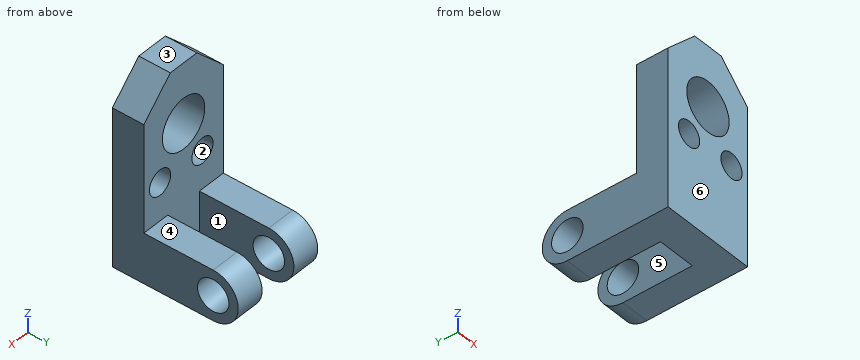
```python
from build123d import *

# Parameters (mm, degrees)
SKETCH2_W           = 30
SKETCH2_H           = 60
BOSS_EXTRUDE1_DEPTH = 10
CHAMFER1_SIZE       = 10
CHAMFER2_SIZE       = 10
SKETCH3_W           = 15.904721494
SKETCH3_H           = 22
BOSS_EXTRUDE2_DEPTH = 9
CUT_EXTRUDE4_REACH  = 56.771
SKETCH5_R           = 8
SKETCH6_R           = 7.952360747
BOSS_EXTRUDE3_DEPTH = 9
CUT_EXTRUDE5_REACH  = 70.795
SKETCH8_R           = 5
CUT_EXTRUDE6_REACH  = 60.421
SKETCH9_R           = 4


with BuildPart() as part:
    # Sketch2 → Boss-Extrude1 (new body)
    with BuildSketch(Plane(origin=(0, 0, 0), x_dir=(1, 0, 0), z_dir=(0, 1, 0))):
        with Locations((-1.70984456, 17.292746114)):
            Rectangle(SKETCH2_W, SKETCH2_H)
    extrude(amount=BOSS_EXTRUDE1_DEPTH)

    # Chamfer1
    chamfer1_edges = [part.edges().sort_by_distance(p)[0] for p in [
        (-16.70984456, 5, 12.707253886),
    ]]
    chamfer(chamfer1_edges, length=CHAMFER1_SIZE)

    # Chamfer2
    chamfer2_edges = [part.edges().sort_by_distance(p)[0] for p in [
        (13.29015544, 5, 12.707253886),
    ]]
    chamfer(chamfer2_edges, length=CHAMFER2_SIZE)

    # Sketch3 → Boss-Extrude2 (add)
    with BuildSketch(Plane(origin=(13.29015544, 0, 0), x_dir=(0, 0, -1), z_dir=(1, 0, 0))):
        with Locations((39.340385367, 21)):
            Rectangle(SKETCH3_W, SKETCH3_H)
    boss_extrude2 = extrude(amount=-BOSS_EXTRUDE2_DEPTH)

    # Sketch5 → Cut-Extrude4 (cut, up to next)
    with BuildSketch(Plane(origin=(0, 10, 0), x_dir=(1, 0, 0), z_dir=(0, 1, 0)), mode=Mode.PRIVATE) as cut_extrude4_sk1:
        with Locations(Location((-1.70984456, 6.38802462, 0), (0, 0, 270))):
            Circle(SKETCH5_R)
    cut_extrude4_tool1 = extrude(cut_extrude4_sk1.sketch, amount=-CUT_EXTRUDE4_REACH, mode=Mode.PRIVATE) & part.part
    add(cut_extrude4_tool1.solids().sort_by_distance((-1.709845, 10, -6.388025))[0], mode=Mode.SUBTRACT)

    # Sketch6 → Boss-Extrude3 (add)
    with BuildSketch(Plane(origin=(13.29015544, 0, 0), x_dir=(0, 0, -1), z_dir=(1, 0, 0))):
        with Locations((39.340385367, 32)):
            Circle(SKETCH6_R)
    boss_extrude3 = extrude(amount=-BOSS_EXTRUDE3_DEPTH)

    # Sketch8 → Cut-Extrude5 (cut, up to next)
    with BuildSketch(Plane(origin=(13.29015544, 0, 0), x_dir=(0, 0, -1), z_dir=(1, 0, 0)), mode=Mode.PRIVATE) as cut_extrude5_sk1:
        with Locations((39.340385367, 32)):
            Circle(SKETCH8_R)
    cut_extrude5_tool1 = extrude(cut_extrude5_sk1.sketch, amount=-CUT_EXTRUDE5_REACH, mode=Mode.PRIVATE) & part.part
    cut_extrude5 = cut_extrude5_tool1.solids().sort_by_distance((13.290155, 32, -39.340385))[0]
    add(cut_extrude5, mode=Mode.SUBTRACT)

    # Mirror6: Boss-Extrude2, Boss-Extrude3, Cut-Extrude5 across plane
    add(boss_extrude2.mirror(Plane.ZY.offset(1.70984456)))
    add(boss_extrude3.mirror(Plane.ZY.offset(1.70984456)))
    add(cut_extrude5.mirror(Plane.ZY.offset(1.70984456)), mode=Mode.SUBTRACT)

    # Sketch9 → Cut-Extrude6 (cut, up to next)
    with BuildSketch(Plane(origin=(0, 10, 0), x_dir=(1, 0, 0), z_dir=(0, 1, 0)), mode=Mode.PRIVATE) as cut_extrude6_sk1:
        with Locations(Location((-8.831623879, 19.34363435, 0), (0, 0, 270))):
            Circle(SKETCH9_R)
    cut_extrude6_tool1 = extrude(cut_extrude6_sk1.sketch, amount=-CUT_EXTRUDE6_REACH, mode=Mode.PRIVATE) & part.part
    # Sketch9 → Cut-Extrude6 (cut, up to next)
    with BuildSketch(Plane(origin=(0, 10, 0), x_dir=(1, 0, 0), z_dir=(0, 1, 0)), mode=Mode.PRIVATE) as cut_extrude6_sk2:
        with Locations(Location((7.168376121, 19.34363435, 0), (0, 0, 270))):
            Circle(SKETCH9_R)
    cut_extrude6_tool2 = extrude(cut_extrude6_sk2.sketch, amount=-CUT_EXTRUDE6_REACH, mode=Mode.PRIVATE) & part.part
    add(cut_extrude6_tool1.solids().sort_by_distance((-8.831624, 10, -19.343634))[0], mode=Mode.SUBTRACT)
    add(cut_extrude6_tool2.solids().sort_by_distance((7.168376, 10, -19.343634))[0], mode=Mode.SUBTRACT)


solid = part.part
```
Design review of the part built by this model. Coordinates are the model's own, in mm. Face numbers are marked on the shaded views. A direction names the side the tool comes from. Give positions to 0.01 mm unless a question says otherwise; leave off trailing zeros. Order: outer loops, then holes, each group sorted by start corner. A loop starts at its lowest first (then second) coordinate and runs counter-clockwise, first axis right, second up. Notation, with made-up numbers: (31, 25.5) - (51, 25.5) arc R20 ccw to (51, 61.5) - close; hole circle Ø5 at (77.25, -28.5). An arc over 180 degrees is marked (long way). Use a Markdown table: item, result. Add a question column.
(1) Mouldability with a two-part tool opening along Z and no side actions: class the marked faces 1, 2 and 3 as +Z half, -Z half, draft (parallel to the pull), parting line (faces both ways), or undercut.
(2) Add section D-D on y = 28.5. Give the boundary of the cut face in (x, z), then the cut area to 3 significant figures.
(3) Wall thickness on probe 1 along X at (y, z) = (16, -37.5); probe 2 along Y at (x, z) = (-0.5, -36); probe 3 along Z at (x, y) = (5.5, 36): over which ranges is each line inside the solid? List them lowest first. Write a range as [from, to].
(4) Add section B-B on y = 12.5. Give the boundary of the cut face in (x, z), then the cut area to 3 significant figures.
(5) Add section A-A on x = -10.5. Give the boundary of the cut face in (y, z), then the cut area to 3 significant figures.
(6) Machinability: for the marked faces 4, 5 and 6, which of the approach directions +Z, -Z, +X, -X, +Y, -Y give a long, thin tool a straight path to every point of the face, cutting with its end or side? Answer none if there is none.
(7) Clearance check with flat-ended pins moving along their axes: P1, Ø4.5, axis at x = 7.5, y = 26, coming from the +Z side; P2, Ø6, axis at x = 8, y = 7.5, coming from the +Z side; P3, Ø1.5, axis at x = 2, z = 4, coming from the +Y side. State where each tip first meets the part, or that it passes through.
(8) Add section C-C on z = -43. Give the boundary of the cut face in (x, y).
Report:
| question | item | result |
|---|---|---|
| 1 | face 1 | draft |
| 1 | face 2 | undercut |
| 1 | face 3 | +Z half |
| 2 | outline | (-16.71, -47.29) - (-7.71, -47.29) - (-7.71, -42.91) - (-16.71, -42.91) - close; (-16.71, -35.77) - (-7.71, -35.77) - (-7.71, -31.39) - (-16.71, -31.39) - close; (4.29, -47.29) - (13.29, -47.29) - (13.29, -42.91) - (4.29, -42.91) - close; (4.29, -35.77) - (13.29, -35.77) - (13.29, -31.39) - (4.29, -31.39) - close |
| 2 | area | 158 mm² |
| 3 | probe 1 | x = [-16.71, -7.71], [4.29, 13.29] |
| 3 | probe 2 | y = [0, 10] |
| 3 | probe 3 | z = [-46.21, -42.34], [-36.34, -32.47] |
| 4 | outline | (-16.71, -47.29) - (-7.71, -47.29) - (-7.71, -31.39) - (-16.71, -31.39) - close; (4.29, -47.29) - (13.29, -47.29) - (13.29, -31.39) - (4.29, -31.39) - close |
| 4 | area | 286 mm² |
| 5 | outline | (0, -47.29) - (32, -47.29) arc R7.95 ccw to (32, -31.39) - (10, -31.39) - (10, -22.98) - (0, -22.98) - close; (0, -15.71) - (10, -15.71) - (10, 8.92) - (0, 8.92) - close; hole circle Ø10 at (32, -39.34) |
| 5 | area | 860 mm² |
| 6 | face 4 | +Z, +X, -X, +Y |
| 6 | face 5 | +Z, -Z, +Y |
| 6 | face 6 | +Z, -Z, +X, -X, -Y |
| 7 | P1 | stops at z = -31.39 |
| 7 | P2 | stops at z = 11 |
| 7 | P3 | stops at y = 10 |
| 8 | outline | (-16.71, 0) - (13.29, 0) - (13.29, 28.59) - (4.29, 28.59) - (4.29, 10) - (-7.71, 10) - (-7.71, 28.59) - (-16.71, 28.59) - close; (-16.71, 35.41) - (-7.71, 35.41) - (-7.71, 39.06) - (-16.71, 39.06) - close; (4.29, 35.41) - (13.29, 35.41) - (13.29, 39.06) - (4.29, 39.06) - close |
